Geometry check sheet. Reference: drawing and pictorial views, mm from the part's lowest x, y, z. A direction names the side the tool comes from. Round coordinates to 2 decimals unless told otherwise and drop trailing zeros. Answer in a Markdown table with one row per item. Add a question column.
1. Set-up check for the marked faces 1 and 2: record each of +Z, -Z, +X, -X, +Y, -Y from which the full face is reachable in a straight line by a thin tool's end or side.
2. Go/stop test with flat-tipped pins: pin 1 Ø3 at (y, z) = (12.7, 3.175) entering from -X; pin 2 Ø3 at (y, z) = (16.5, 3) entering from +X (1 decimal); pin 3 Ø1.9 at (x, z) = (15.5, 3.5) entering from +Y (1 decimal); pin 4 Ø1 at (x, y) = (15.5, 12) entering from -Z. Record where each tip stops, or that it passes through.
3. Material ranges on probe 1 along Y at (x, z) = (9.75, 5) (1 decimal); probe 2 along Y at (x, z) = (5.25, 3), recorded low to high.
4. Draft check along Y on the marked faces 3, 4, 5 and 6. Enter one of: pulls with the +Y half, pulls with the -Y half, needs draft (parallel to the pull), parting line crosses it, or undercut.
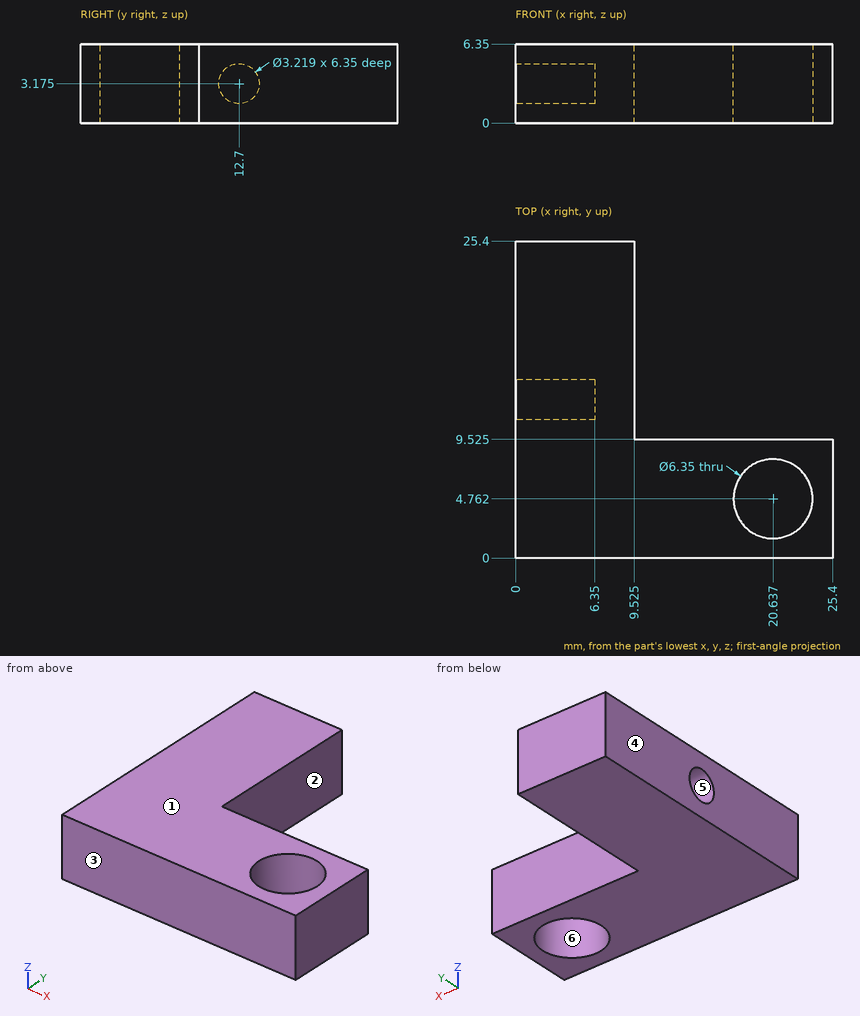
Geometry check:
| question | item | result |
|---|---|---|
| 1 | face 1 | +Z, +X, -X, +Y, -Y |
| 1 | face 2 | +Z, -Z, +X, +Y |
| 2 | pin 1 | stops at x = 6.35 |
| 2 | pin 2 | stops at x = 9.5 |
| 2 | pin 3 | stops at y = 9.5 |
| 2 | pin 4 | passes through |
| 3 | probe 1 | y = 0 to 9.5 |
| 3 | probe 2 | y = 0 to 11.1, 14.3 to 25.4 |
| 4 | face 3 | pulls with the -Y half |
| 4 | face 4 | needs draft |
| 4 | face 5 | undercut |
| 4 | face 6 | undercut |
